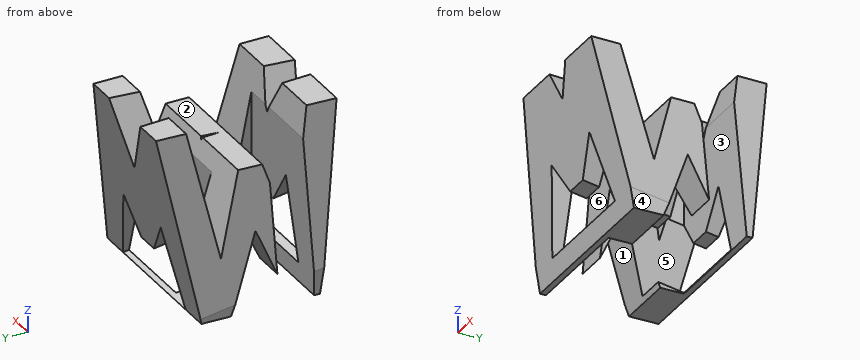
```python
from build123d import *

# Parameters (mm, degrees)
F0_W     = 38.1
F0_H     = 38.0999925736
F1_DEPTH = 38.1
F4_DEPTH = 38.1
F6_DEPTH = 38.1
F7_W     = 25.4
F7_H     = 7.62
F8_DEPTH = 38.1


with BuildPart() as f1:
    # F0 (on Front) → F1 (new body)
    with BuildSketch(Plane.XZ):
        with Locations((19.05, 19.0499962868)):
            Rectangle(F0_W, F0_H)
    extrude(amount=F1_DEPTH)

    # F3 (on face) → F4 (cut)
    with BuildSketch(Plane.YZ.offset(38.1)):
        Polygon((-6.35, 38.0999925736), (-31.75, 38.0999925736), (-26.67, 12.4402772635), (-21.59, 28.575), (-16.51, 28.575), (-11.43, 11.9197117337), align=None)
        Polygon((-31.75, 0), (-38.1, 38.0999925736), (-38.1, 0), align=None)
        Polygon((-19.05, 15.875), (-25.4, 0), (-12.7, 0), align=None)
        Polygon((0, 0), (0, 38.0999925736), (-6.35, 0), align=None)
    extrude(amount=-F4_DEPTH, mode=Mode.SUBTRACT)

    # F5 (on face) → F6 (cut)
    with BuildSketch(Plane(origin=(0, -6.1783783133, 1.0297299196), x_dir=(-1, 0, 0), z_dir=(0, 0.9863939186, -0.1643990185))):
        Polygon((-26.67, 15.0061463937), (-31.75, -1.0439337674), (-6.35, -1.0439337674), (-11.43, 15.1532115415), (-16.51, 7.6999627054), (-21.59, 7.6999627054), align=None)
        Polygon((-38.1, -1.0439337674), (-31.75, 37.5816009747), (-38.1, 37.5816009747), align=None)
        Polygon((-12.7, 37.5816009747), (-25.4, 37.5816009747), (-19.05, 24.8909872025), align=None)
        Polygon((0, 37.5816009747), (-6.35, 37.5816009747), (0, 0), align=None)
    extrude(amount=-F6_DEPTH, mode=Mode.SUBTRACT)

    # F7 (on offset) → F8 (cut)
    with BuildSketch(Plane.XY.offset(38.1)):
        with Locations((25.4, -11.43)):
            Rectangle(F7_W, F7_H)
        with Locations((12.7, -26.67)):
            Rectangle(F7_W, F7_H)
    extrude(amount=-F8_DEPTH, mode=Mode.SUBTRACT)


solid = f1.part
```
Input: part model. Units: mm. Frame: model coordinates. Face numbers are marked on the shaded views. A direction names the side the tool comes from. Round coordinates to 2 decimals unless told otherwise and drop trailing zeros. Loops run counter-clockwise (first coordinate to the right, second up) from the corner with the lowest first, then second, coordinate; pieces in that order, holes last. Notation, with made-up numbers: (81, -1) -> (111, -1) arc R9 ccw to (111, 5) -> close; hole circle Ø7 at (7.25, -31). An arc over 180 degrees is marked (long way). One line per item, written item: value.
(1) Mould query, pull axis X, two halves, no side actions, for the marked faces 4, 5 and 6. Classes: pulls with the +X half, pulls with the -X half, needs draft (parallel to the pull), parting line crosses it, or undercut.
Geometry check:
face 4: pulls with the +X half
face 5: undercut
face 6: needs draft
(2) Material intervals for line 1 (Y direction, x = 30, z = 23); line 2 (Y direction, x = 32, z = 15.5); line 3 (Y direction, x = 20, z = 18.5), sorted ascending. Write a range as [from, to].
Geometry check:
line 1: [-35.58, -28.76], [-23.35, -15.24], [-7.62, -2.52]
line 2: [-34.33, -27.28], [-25.71, -19.2], [-18.9, -15.24], [-7.62, -3.77]
line 3: [-34.83, -30.48], [-22.86, -15.24], [-7.62, -3.27]
(3) Section A-A (z = 22.5). Return the cut outline in (x, y) (3 decimals).
Geometry check:
outline: (2.764, -35.5) -> (35.239, -35.5) -> (35.054, -28.662) -> (25.4, -28.662) -> (25.4, -30.48) -> (2.903, -30.48) -> close; (3.115, -22.86) -> (25.4, -22.86) -> (25.4, -23.503) -> (34.915, -23.503) -> (34.692, -15.24) -> (12.7, -15.24) -> (12.7, -14.657) -> (3.343, -14.657) -> close; (3.49, -9.377) -> (12.7, -9.377) -> (12.7, -7.62) -> (34.486, -7.62) -> (34.35, -2.6) -> (3.678, -2.6) -> close
(4) Pin query (flat end, axial travel): pin 1 (6 mm diameter, centred on x = 10, z = 15.5, fed in from -Y); pin 2 (10 mm diameter, centred on x = 5, z = 34, fed in from -Y); pin 3 (3.5 mm diameter, centred on y = -9, z = 23, fed in from +X); pin 4 (8 mm diameter, centred on y = -16, z = 6.5, fed in from -X). Return the tip coordinate at first contact, or that it passes through.
Geometry check:
pin 1: y = -34.83
pin 2: y = -38.1
pin 3: x = 34.58
pin 4: x = 0.13
(5) Section B-B (z = 33). Return the cut outline in (x, y), plus the area to 3 significant figures.
Geometry check:
outline: (4.47, -37.25) -> (18.28, -37.25) -> (17.75, -30.74) -> (4.65, -30.74) -> close; (5.3, -7.34) -> (15.82, -7.34) -> (15.29, -0.85) -> (5.48, -0.85) -> close; (19.82, -37.25) -> (33.58, -37.25) -> (33.41, -30.74) -> (20.35, -30.74) -> close; (22.28, -7.34) -> (32.78, -7.34) -> (32.6, -0.85) -> (22.81, -0.85) -> close
area: 307 mm2
(6) Set-up query: the marked faces 1, 2 and 3. Return all of +Z, -Z, +X, -X, +Y, -Y with unobstructed straight access to the full face (end or side cutting, diameter ignored); none if empty.
Geometry check:
face 1: -Z, +X, -X
face 2: +Z, +X, -X
face 3: +Z, -Z, +X
